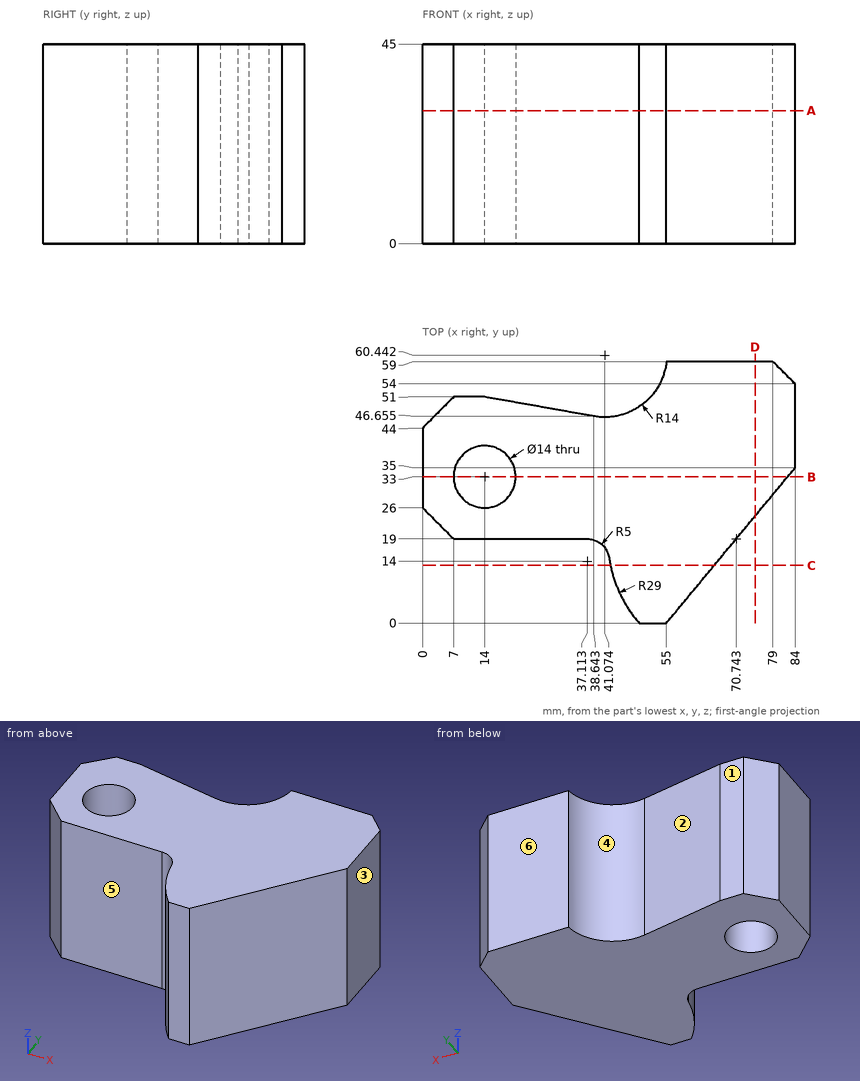
Drawing for the job (mm, zero at the part's lowest x, y, z). A direction names the side the tool comes from. Coordinates: 2 decimals unless noted, no trailing zeros. Order: outer loops, then holes, each group sorted by start corner. A loop starts at its lowest first (then second) coordinate and runs counter-clockwise, first axis right, second up. Notation, with made-up numbers: (62, -31.5) - (76, -31.5) arc R27 cw to (76, -0.5) - close; hole circle Ø11 at (86.25, 68.25). An arc over 180 degrees is marked (long way). Use a Markdown table: item, result. Add a question column.
(1) Drill centre lines: line 1 along Y through (x, z) = (14, 13); line 2 along Y through (x, z) = (10, 38.5) (1 decimal); line 3 along X through (y, z) = (33, 16.5) (1 decimal). Where is each one in solid material? Low to high. Write a range as [from, to].
(2) Saw through at B-B (y = 33). Give the cut face in (x, z).
(3) Saw through at C-C (y = 13). Give the cut face in (x, z), then the cut area to 3 significant figures.
(4) Pull direction X, two halves, no side cores. Call the marked faces 1, 2, 3 and 4: +X half, -X half, draft (parallel to the pull), parting line (faces both ways), or undercut.
(5) Flat gauge pins, fed straight in: pin 1 (7.5 mm diameter, centred on x = 10, z = 24, fed in from +Y); pin 2 (1.5 mm diameter, centred on x = 36.5, z = 40.5, fed in from -Y); pin 3 (12 mm diameter, centred on y = 21, z = 22.5, fed in from +X). Where does each tip first touch, or does it go through?
(6) Which spindle directions (+Z, -Z, +X, -X, +Y, -Y) get a long thin tool onto all of the face, cutting with end or side? Do the marked faces 5 and 6. Say none if no direction does.
(7) Saw through at A-A (z = 30). Give the cut face in (x, y) (1 decimal).
(8) Saw through at D-D (x = 75). Give the cut face in (y, z), then the cut area to 3 significant figures.
Solved:
| question | item | result |
|---|---|---|
| 1 | line 1 | y = [19, 26], [40, 51] |
| 1 | line 2 | y = [19, 27.3], [38.7, 51] |
| 1 | line 3 | x = [0, 7], [21, 82.3] |
| 2 | outline | (0, 0) - (7, 0) - (7, 45) - (0, 45) - close; (21, 0) - (82.34, 0) - (82.34, 45) - (21, 45) - close |
| 3 | outline | (42.37, 0) - (65.77, 0) - (65.77, 45) - (42.37, 45) - close |
| 3 | area | 1,050 mm² |
| 4 | face 1 | draft |
| 4 | face 2 | undercut |
| 4 | face 3 | +X half |
| 4 | face 4 | undercut |
| 5 | pin 1 | stops at y = 51 |
| 5 | pin 2 | stops at y = 19 |
| 5 | pin 3 | stops at x = 77.37 |
| 6 | face 5 | +Z, -Z, -X, -Y |
| 6 | face 6 | +Z, -Z, +X, -X, +Y |
| 7 | outline | (0, 26) - (7, 19) - (37.1, 19) arc R5 cw to (42.1, 14.7) arc R29 ccw to (48.8, 0) - (55, 0) - (84, 35) - (84, 54) - (79, 59) - (55, 59) arc R14 cw to (38.6, 46.7) - (14, 51) - (7, 51) - (0, 44) - close; hole circle Ø14 at (14, 33) |
| 8 | outline | (24.14, 0) - (59, 0) - (59, 45) - (24.14, 45) - close |
| 8 | area | 1,570 mm² |
